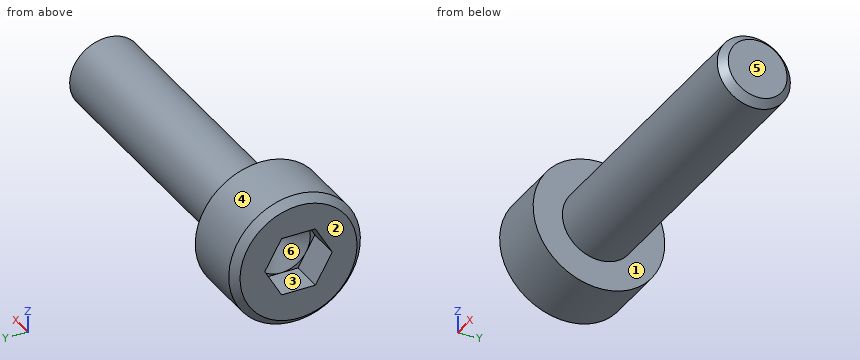
```python
from build123d import *

# Parameters (mm, degrees)
CUT_EXTRUDE_1_DEPTH = 1.1


with BuildPart() as part:
    # Sketch 1 → Revolve 1 (revolve)
    with BuildSketch(Plane.XY, mode=Mode.PRIVATE) as revolve_1_sk:
        Polygon((-2.36, 0), (-2.36, 2), (-2.11, 2.25), (0, 2.25), (0, 1.25), (9.7565, 1.25), (10, 1.0065), (10, 0), align=None)
    revolve(revolve_1_sk.sketch.rotate(Axis((10, 0, 0), (-1, 0, 0)), 270), axis=Axis((10, 0, 0), (-1, 0, 0)))

    # Sketch 2 → Cut-Extrude 1 (cut)
    with BuildSketch(Plane(origin=(-2.36, 0, 0), x_dir=(0, 0, -1), z_dir=(1, 0, 0))):
        Polygon((-1, 0.577350269), (-1, -0.577350269), (0, -1.154700538), (1, -0.577350269), (1, 0.577350269), (0, 1.154700538), align=None)
    extrude(amount=CUT_EXTRUDE_1_DEPTH, mode=Mode.SUBTRACT)

    # Sketch 3 → Cut-Revolve 1 (revolve, cut)
    with BuildSketch(Plane.XY, mode=Mode.PRIVATE) as cut_revolve_1_sk:
        Polygon((-1.26, 0), (-1.26, 1), (-0.682649731, 0), align=None)
    revolve(cut_revolve_1_sk.sketch.rotate(Axis((-0.682649731, 0, 0), (-1, 0, 0)), 270), axis=Axis((-0.682649731, 0, 0), (-1, 0, 0)), mode=Mode.SUBTRACT)


solid = part.part
```
For this review, take the finished solid that the model builds, in its own axes (mm). Face numbers are marked on the shaded views. A direction names the side the tool comes from. Coordinates: 2 decimals unless noted, no trailing zeros. Write each loop counter-clockwise with the first axis right and the second up, starting at its lowest first coordinate (ties: lowest second). Pieces come first, ordered by that corner, then holes.
(1) For pin 1 Ø1.5 at (x, y) = (-1, 1) entering from +Z; pin 2 Ø1.5 at (x, y) = (1.5, 0) entering from +Z, all flat-tipped, find the tip position at first contact; note any pin that passes through.
(2) Wall thickness on probe 1 along X at (y, z) = (-0.05, -1.85); probe 2 along Y at (x, z) = (5.25, 0); probe 3 along Y at (x, z) = (4, -0.55): over which ranges is each line inside the solid? List them lowest first.
(3) Add section A-A on x = 9.5. Give the boundary of the cut face in (y, z), then the cut area to 3 significant figures.
(4) Tool access review of the marked faces 1, 2 and 3: name each direction out of +Z, -Z, +X, -X, +Y, -Y from which nothing blocks a thin tool from reaching the whole face with its end or side.
(5) The part is to be moulded in two halves that separate along Y. For the marked faces 4, 5 and 6, say which applies: +Y half, -Y half, draft (parallel to the pull), parting line (faces both ways), or undercut.
Answer sheet:
1. pin 1: stops at z = 2.24
1. pin 2: stops at z = 1.25
2. probe 1: x = -2.36 to 0
2. probe 2: y = -1.25 to 1.25
2. probe 3: y = -1.12 to 1.12
3. outline: circle Ø2.5 at (0, 0)
3. area: 4.91 mm2
4. face 1: +X
4. face 2: +Z, -Z, -X, +Y, -Y
4. face 3: -X
5. face 4: parting line
5. face 5: draft
5. face 6: undercut
